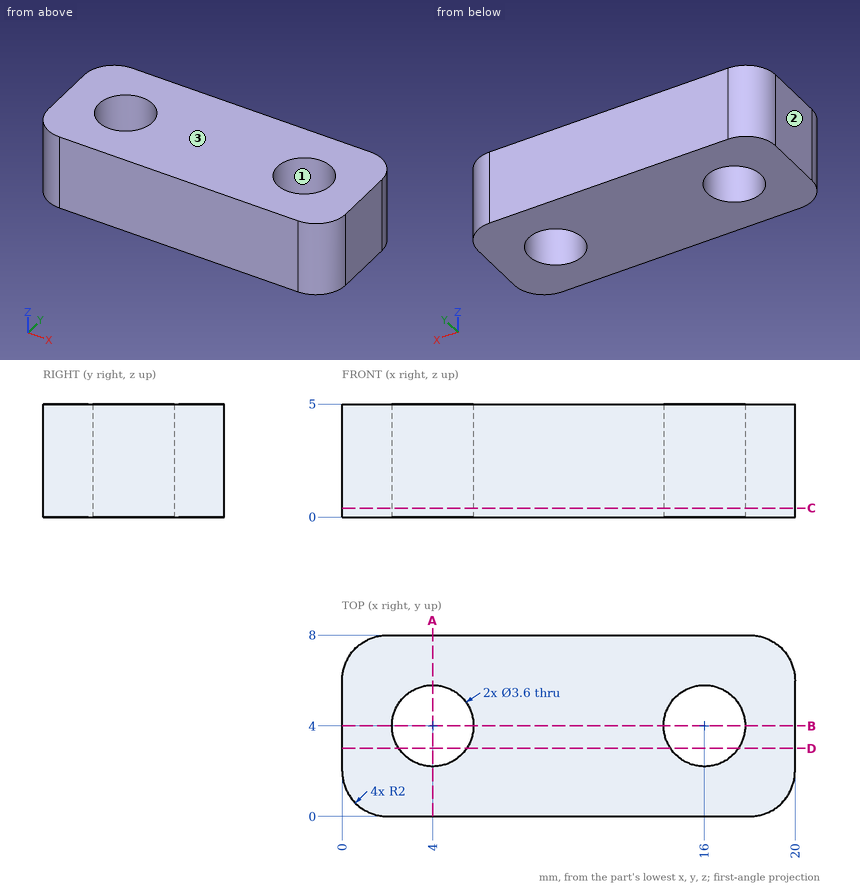
Study the drawing (mm; zero at the part's minimum x, y, z) and answer. Round coordinates to 2 decimals unless told otherwise and drop trailing zeros. Write each loop counter-clockwise with the first axis right and the second up, starting at its lowest first coordinate (ties: lowest second). Pieces come first, ordered by that corner, then holes.
Q1. Straight lines are drawn through the part: line 1 (Y direction, x = 4, z = 2.55); line 2 (X direction, y = 3.25, z = 1.1); line 3 (X direction, y = 2.5, z = 4.7). For each, find the intervals that lie inside material, in ascending order.
Values:
line 1: y = 0 to 2.2, 5.8 to 8
line 2: x = 0 to 2.36, 5.64 to 14.36, 17.64 to 20
line 3: x = 0 to 3.01, 4.99 to 15.01, 16.99 to 20
Q2. Find section B-B on y = 4. Determine the outline of the cut face in (x, z), and give its area (3 significant figures).
Values:
outline: (0, 0) - (2.2, 0) - (2.2, 5) - (0, 5) - close; (5.8, 0) - (14.2, 0) - (14.2, 5) - (5.8, 5) - close; (17.8, 0) - (20, 0) - (20, 5) - (17.8, 5) - close
area: 64.0 mm2
Q3. Find section A-A on x = 4. Determine the outline of the cut face in (y, z), and give its area (3 significant figures).
Values:
outline: (0, 0) - (2.2, 0) - (2.2, 5) - (0, 5) - close; (5.8, 0) - (8, 0) - (8, 5) - (5.8, 5) - close
area: 22.0 mm2
Q4. The mould has two halves that part along X. Classify the marked faces 1, 2 and 3: released by +X, released by -X, zero draft, split by the parting line, or undercut.
Values:
face 1: undercut
face 2: released by -X
face 3: zero draft
Q5. Find section D-D on y = 3. Determine the outline of the cut face in (x, z), and give its area (3 significant figures).
Values:
outline: (0, 0) - (2.5, 0) - (2.5, 5) - (0, 5) - close; (5.5, 0) - (14.5, 0) - (14.5, 5) - (5.5, 5) - close; (17.5, 0) - (20, 0) - (20, 5) - (17.5, 5) - close
area: 70.1 mm2
Q6. Find section C-C on z = 0.4. Determine the outline of the cut face in (x, y), and give its area (3 significant figures).
Values:
outline: (0, 2) arc R2 ccw to (2, 0) - (18, 0) arc R2 ccw to (20, 2) - (20, 6) arc R2 ccw to (18, 8) - (2, 8) arc R2 ccw to (0, 6) - close; hole circle Ø3.6 at (4, 4); hole circle Ø3.6 at (16, 4)
area: 136 mm2
